Design review of the part built by this model. Coordinates are the model's own, in mm. Face numbers are marked on the shaded views. A direction names the side the tool comes from. Round coordinates to 2 decimals unless told otherwise and drop trailing zeros. Order: outer loops, then holes, each group sorted by start corner. A loop starts at its lowest first (then second) coordinate and runs counter-clockwise, first axis right, second up. Notation, with made-up numbers: (-15.5, -18) - (4.5, -18) arc R27 ccw to (4.5, 0) - close; hole circle Ø4 at (-13, -7). An arc over 180 degrees is marked (long way). Answer as a JSON object with one key per item and string values. Group by question number.
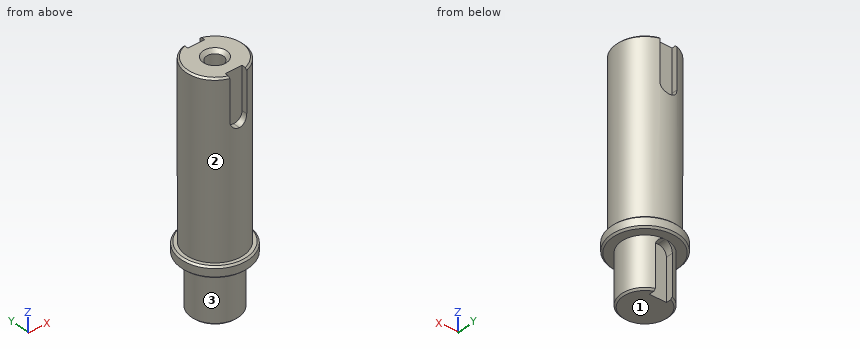
from build123d import *

# Parameters (mm, degrees)
SKETCH_1_R               = 7
EXTRUDE_1_DEPTH          = 15
SKETCH_3_R               = 10
EXTRUDE_2_DEPTH          = 3.3
SKETCH_4_R               = 8.5
EXTRUDE_3_DEPTH          = 51
SKETCH_6_W               = 5
SKETCH_6_H               = 2.626010101
CUT_EXTRUDE_1_DEPTH      = 15
FILLET_1_R               = 2.5
SKETCH_7_R               = 2.5
CUT_EXTRUDE_2_DEPTH      = 15
SKETCH_8_W               = 5
SKETCH_8_H               = 2.5
CUT_EXTRUDE_3_DEPTH      = 15
FILLET_2_R               = 2.5
CHAMFER_1_SIZE           = 1
CHAMFER_2_SIZE           = 0.5
CHAMFER_3_SIZE           = 0.5
PATTERN_CIRCULAR_1_COUNT = 2
FILLET_3_R               = 2.5


with BuildPart() as part:
    # 草图1 → 拉伸1 (new body)
    with BuildSketch(Plane.XY):
        Circle(SKETCH_1_R)
    extrude(amount=EXTRUDE_1_DEPTH)

    # 草图3 → 拉伸2 (add)
    with BuildSketch(Plane.XY.offset(15)):
        Circle(SKETCH_3_R)
    extrude(amount=EXTRUDE_2_DEPTH)

    # 草图4 → 拉伸3 (add)
    with BuildSketch(Plane.XY.offset(18.3)):
        Circle(SKETCH_4_R)
    extrude(amount=EXTRUDE_3_DEPTH)

    # 草图6 → 切除-拉伸1 (cut)
    with BuildSketch(Plane.XY.offset(69.3)):
        with Locations((0, 7.813005051)):
            Rectangle(SKETCH_6_W, SKETCH_6_H)
    cut_extrude_1 = extrude(amount=-CUT_EXTRUDE_1_DEPTH, mode=Mode.SUBTRACT)

    # 圆角1
    fillet_1_edges = [part.edges().sort_by_distance(p)[0] for p in [
        (-2.5, 7.312019202, 54.3),
        (2.5, 7.312019202, 54.3),
    ]]
    fillet(fillet_1_edges, radius=FILLET_1_R - 0.0001)  # a hair under: the kernel refuses the full size

    # 草图7 → 切除-拉伸2 (cut)
    with BuildSketch(Plane.XY.offset(69.3)):
        Circle(SKETCH_7_R)
    extrude(amount=-CUT_EXTRUDE_2_DEPTH, mode=Mode.SUBTRACT)

    # 草图8 → 切除-拉伸3 (cut)
    with BuildSketch(Plane(origin=(0, 0, 0), x_dir=(-1, 0, 0), z_dir=(0, 0, -1))):
        with Locations((0, 5.75)):
            Rectangle(SKETCH_8_W, SKETCH_8_H)
    extrude(amount=-CUT_EXTRUDE_3_DEPTH, mode=Mode.SUBTRACT)

    # 圆角2
    fillet_2_edges = [part.edges().sort_by_distance(p)[0] for p in [
        (-2.5, 5.519174208, 15),
        (2.5, 5.519174208, 15),
    ]]
    fillet(fillet_2_edges, radius=FILLET_2_R - 0.0001)  # a hair under: the kernel refuses the full size

    # 倒角1
    chamfer_1_edges = [part.edges().sort_by_distance(p)[0] for p in [
        (-2.5, 0, 69.3),
    ]]
    chamfer(chamfer_1_edges, length=CHAMFER_1_SIZE)

    # 倒角2
    chamfer_2_edges = [part.edges().sort_by_distance(p)[0] for p in [
        (-5.049752469, -6.837397166, 69.3),
        (-10, 0, 15),
        (-10, 0, 18.3),
    ]]
    chamfer(chamfer_2_edges, length=CHAMFER_2_SIZE)

    # 倒角3
    chamfer_3_edges = [part.edges().sort_by_distance(p)[0] for p in [
        (0, -7, 0),
    ]]
    chamfer(chamfer_3_edges, length=CHAMFER_3_SIZE)

    # 阵列(圆周)1: 切除-拉伸1 ×2 about axis
    pattern_circular_1_axis = Axis((0, 0, 0), (0, 0, 1))
    for i in range(1, PATTERN_CIRCULAR_1_COUNT):
        add(cut_extrude_1.rotate(pattern_circular_1_axis, i * 360 / PATTERN_CIRCULAR_1_COUNT), mode=Mode.SUBTRACT)

    # 圆角3
    fillet_3_edges = [part.edges().sort_by_distance(p)[0] for p in [
        (-2.5, -7.312019202, 54.3),
        (2.5, -7.312019202, 54.3),
    ]]
    fillet(fillet_3_edges, radius=FILLET_3_R - 0.0001)  # a hair under: the kernel refuses the full size


solid = part.part
1. Clearance check with flat-ended pins moving along their axes: P1, Ø5.5, axis at x = 0, y = 0, coming from the +Z side; P2, Ø5.5, axis at x = -3.5, y = 2, coming from the -Z side; P3, Ø6, axis at x = 7, z = 44.5, coming from the -Y side; P4, Ø5.5, axis at x = 1, z = 65, coming from the -Y side. State where each tip first meets the part, or that it passes through.
2. To check wall thickness, follow line 1 (Y direction, x = 0, z = 58.25); line 2 (Z direction, x = 7.75, y = 0); line 3 (Z direction, x = 0.25, y = 7). State the ranges of each line that lie inside material, in increasing order. Write a range as from..to.
3. Tool access review of the marked faces 1, 2 and 3: name each direction out of +Z, -Z, +X, -X, +Y, -Y from which nothing blocks a thin tool from reaching the whole face with its end or side.
4. Take a section at A-A, the plane z = 24. Give the boundary of the cut face in (x, y).
Response values:
{
 "1": {"P1": "z = 68.55", "P2": "z = 0", "P3": "y = -7.5", "P4": "y = -8.12"},
 "2": {"line 1": "-6.5..-2.5, 2.5..6.5", "line 2": "15..69.3", "line 3": "15..54.31"},
 "3": {"face 1": "-Z, +X, -X, +Y, -Y", "face 2": "+Z", "face 3": "-Z"},
 "4": {"outline": "circle Ø17 at (0, 0)"}
}
